Autodesk Inventor part; units mm, degrees
ref_plane "YZ Plane" through (0, 0, 0) normal (1, 0, 0) x (0, 1, 0)
ref_plane "XZ Plane" through (0, 0, 0) normal (0, 1, 0) x (-1, 0, 0)
ref_plane "XY Plane" through (0, 0, 0) normal (0, 0, 1) x (1, 0, 0)
sketch "Sketch1" plane through (0, 0, 0) normal (0, 0, 1) x (1, 0, 0)
  line L0 (0, -5.6) -> (0, 5.6) construction
  line L1 (-16.8, 0) -> (16.8, 0) construction
  line L2 (8, 4) -> (-8, 4)
  arc A0 (-8, 4) -> (-8, -4) centre (-8, 0) ccw
  line L3 (-8, -4) -> (8, -4)
  arc A1 (8, -4) -> (8, 4) centre (8, 0) ccw
  circle A2 centre (0, 0) radius 2.75
  circle A3 centre (0, 0) radius 2.4
  point P0 (0, 4)
  dimension "d0" = 24
  dimension "d1" = 8
  dimension "d27" = 4.8
  dimension "d28" = 5.5
sketch "Sketch6" plane through (0, 0, 0) normal (0, 0, 1) x (1, 0, 0)
  arc A0 (-8, 4) -> (-8, -4) centre (-8, 0) ccw construction
  arc A1 (8, -4) -> (8, 4) centre (8, 0) ccw construction
  circle A2 centre (-8, 0) radius 2.3
  circle A3 centre (8, 0) radius 2.3
  line L0 (-10.1564, 0.8) -> (-8.8, 0.8)
  line L1 (-8.8, 0.8) -> (-8.8, 2.1564)
  line L2 (-7.2, 2.1564) -> (-7.2, 0.8)
  line L3 (-7.2, 0.8) -> (-5.8436, 0.8)
  line L4 (-5.8436, -0.8) -> (-7.2, -0.8)
  line L5 (-7.2, -0.8) -> (-7.2, -2.1564)
  line L6 (-8.8, -2.1564) -> (-8.8, -0.8)
  line L7 (-8.8, -0.8) -> (-10.1564, -0.8)
  line L8 (5.8436, 0.8) -> (7.2, 0.8)
  line L9 (8.8, 0.8) -> (10.1564, 0.8)
  line L10 (8.8, 2.1564) -> (8.8, 0.8)
  line L11 (8.8, -0.8) -> (8.8, -2.1564)
  line L12 (7.2, 2.1564) -> (7.2, 0.8)
  line L13 (7.2, -0.8) -> (7.2, -2.1564)
  line L14 (10.1564, -0.8) -> (8.8, -0.8)
  line L15 (7.2, -0.8) -> (5.8436, -0.8)
  dimension "d29" = 4.6
  dimension "d30" = 1.6
extrude "Extrusion1" add sketch "Sketch1" along normal mid plane 4 contours A1 L3 A0 L2 | A2 | A3
extrude "Extrusion2" cut sketch "Sketch1" along normal through all both and the other way through all contours A3
sketch "Sketch2" plane through (0, 0, 2) normal (0, 0, 1) x (1, 0, 0)
  circle A0 centre (0, 0) radius 2.75
extrude "Extrusion3" cut sketch "Sketch2" against normal blind 0.5333
sketch "Sketch3" plane through (0, 0, -2) normal (0, 0, -1) x (-1, 0, 0)
  circle A0 centre (0, 0) radius 2.75
extrude "Extrusion4" cut sketch "Sketch3" against normal blind 0.5333
extrude "Extrusion7" cut sketch "Sketch6" along normal through all both and the other way through all contours A2 L4 L5 L6 L7 L0 L1 L2 L3 | A3 L14 L11 L13 L15 L8 L12 L10 L9
sketch "Sketch4" plane through (0, 0, 2) normal (0, 0, 1) x (1, 0, 0)
  circle A0 centre (-8, 0) radius 2.3 construction
  circle A1 centre (8, 0) radius 2.3 construction
  arc A2 (5.9892, 3.3333) -> (5.9892, -3.3333) centre (8, 0) ccw
  line L0 (2.0108, 3.3333) -> (5.9892, 3.3333)
  line L1 (5.9892, -3.3333) -> (2.0108, -3.3333)
  arc A3 (-5.9892, -3.3333) -> (-5.9892, 3.3333) centre (-8, 0) ccw
  line L2 (-5.9892, 3.3333) -> (-2.0108, 3.3333)
  line L3 (-5.9892, -3.3333) -> (-2.0108, -3.3333)
  arc A4 (2.0108, -3.3333) -> (2.0108, 3.3333) centre (0, 0) ccw
  arc A5 (-2.0108, 3.3333) -> (-2.0108, -3.3333) centre (0, 0) ccw
  circle A6 centre (0, 0) radius 2.75 construction
  dimension "d33" = 6.6667
  dimension "d35" = 1.1429
extrude "Extrusion5" cut sketch "Sketch4" against normal blind 0.5333
sketch "Sketch7" plane through (0, 0, -2) normal (0, 0, -1) x (-1, 0, 0)
  arc A0 (5.9892, 3.3333) -> (5.9892, -3.3333) centre (8, 0) ccw
  line L0 (5.9892, -3.3333) -> (2.0108, -3.3333)
  arc A1 (2.0108, -3.3333) -> (2.0108, 3.3333) centre (0, 0) ccw
  line L1 (2.0108, 3.3333) -> (5.9892, 3.3333)
  arc A2 (-2.0108, 3.3333) -> (-2.0108, -3.3333) centre (0, 0) ccw
  line L2 (-2.0108, -3.3333) -> (-5.9892, -3.3333)
  arc A3 (-5.9892, -3.3333) -> (-5.9892, 3.3333) centre (-8, 0) ccw
  line L3 (-5.9892, 3.3333) -> (-2.0108, 3.3333)
extrude "Extrusion8" cut sketch "Sketch7" against normal blind 0.5333
equation "\"d1\" = width_standard"
equation "\"d2\" = 0.5 * width_standard"
equation "\"d6\" = 0.333333 * height_standard"
equation "\"d13\" = 0.0555556 * height_standard"
equation "\"d15\" = 0.0555556 * height_standard"
equation "\"d33\" = 0.833333 * width_standard"
equation "\"d20\" = 0.0555556 * height_standard"
equation "\"d36\" = 0.0555556 * height_standard"
equation "\"width_standard\" = 8"
equation "\"height_standard\" = 9.6"
properties part number "LEGO Brick 32017" material "Steel"
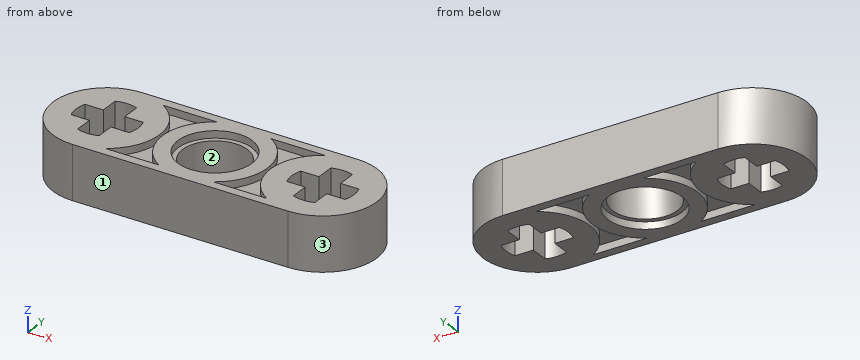
Can you work these out from the model? Positions are in its coordinate system, mm. Face numbers are marked on the shaded views. Round coordinates to 2 decimals unless told otherwise and drop trailing zeros. Loops run counter-clockwise (first coordinate to the right, second up) from the corner with the lowest first, then second, coordinate; pieces in that order, holes last. Notation, with made-up numbers: M -14.75,82 L 44.25,82 A29 cw 44.25,110 Z; hole C 84.25,-31 d10. An arc over 180 degrees is marked long. Write item = value, one per line. Start each with the question number.
(1) I'm going to push flat-ended pins straight in: P1, Ø0.7, axis at x = -9.5, z = 0.5, coming from the -Y side; P2, Ø0.7, axis at y = -2, z = 1, coming from the +X side; P3, Ø1.5, axis at y = 1.5, z = 0, coming from the +X side; P4, Ø1.6, axis at x = 0, y = -1, coming from the +Z side. Where does each tip first touch, or does it pass through?
(2) I need wall thicknesses on line 1 along Y through (x, z) = (0, 1.7); line 2 along X through (y, z) = (-1.25, -1.1); line 3 along Y through (x, z) = (0, 0.05). Which ranges of each line are inside material? Lowest first, please.
(3) Suppose I cut it at A-A on z = 0.3. Give the number of separate pieces and of enclosed holes in the cut face, plus the area to 3 significant figures.
(4) If we mould it in two halves opening along X, with no side actions, what happens to the marked faces 1, 2 and 3? For each: released by +X, released by -X, zero draft, split by the parting line, or undercut.
(5) Suppose I cut it at B-B on x = 0. Write out the boundary of the cut face in (y, z), plus the area to 3 significant figures.
Answer block:
q1.P1 = -3.83
q1.P2 = 11.64
q1.P3 = 11.93
q1.P4 = through
q2.line_1 = -4 to -2.75, 2.75 to 4
q2.line_2 = -11.8 to -8.8, -7.2 to -2.05, 2.05 to 7.2, 8.8 to 11.8
q2.line_3 = -4 to -2.4, 2.4 to 4
q3.separate_pieces = 1
q3.enclosed_holes = 3
q3.area = 136 mm²
q4.face_1 = zero draft
q4.face_2 = undercut
q4.face_3 = released by +X
q5.outline = M -4,-2 L -2.75,-2 L -2.75,-1.47 L -2.4,-1.47 L -2.4,1.47 L -2.75,1.47 L -2.75,2 L -4,2 Z; M 2.4,-1.47 L 2.75,-1.47 L 2.75,-2 L 4,-2 L 4,2 L 2.75,2 L 2.75,1.47 L 2.4,1.47 Z
q5.area = 12.1 mm²
